Verification items for the finished model (mm, model axes). Round coordinates to 2 decimals unless told otherwise and drop trailing zeros. Loops run counter-clockwise (first coordinate to the right, second up) from the corner with the lowest first, then second, coordinate; pieces in that order, holes last. Notation, with made-up numbers: M 13.25,10 L 32.25,10 A35 cw 32.25,45 Z; hole C 25.25,-21 d10. An arc over 180 degrees is marked long. One line per item, written item: value.
Autodesk Inventor part; units mm, degrees
ref_plane "YZ Plane" through (0, 0, 0) normal (1, 0, 0) x (0, 1, 0)
ref_plane "XZ Plane" through (0, 0, 0) normal (0, 1, 0) x (-1, 0, 0)
ref_plane "XY Plane" through (0, 0, 0) normal (0, 0, 1) x (1, 0, 0)
sketch "Sketch1" plane through (0, 0, 0) normal (0, 0, 1) x (1, 0, 0)
  line L0 (-7.5, 73) -> (7.5, 73)
  line L1 (7.5, 73) -> (7.5, 70)
  line L2 (-7.5, 70) -> (-7.5, 73)
  line L3 (-40.4145, 70) -> (-7.5, 70)
  line L4 (7.5, 70) -> (40.4145, 70)
  line L5 (-66.9699, 30.0048) -> (-59.4699, 42.9952)
  line L6 (-59.4699, 42.9952) -> (-56.8718, 41.4952)
  line L7 (-64.3718, 28.5048) -> (-66.9699, 30.0048)
  line L8 (-59.4699, -42.9952) -> (-66.9699, -30.0048)
  line L9 (-66.9699, -30.0048) -> (-64.3718, -28.5048)
  line L10 (-56.8718, -41.4952) -> (-59.4699, -42.9952)
  line L11 (7.5, -73) -> (-7.5, -73)
  line L12 (-7.5, -73) -> (-7.5, -70)
  line L13 (7.5, -70) -> (7.5, -73)
  line L14 (66.9699, -30.0048) -> (59.4699, -42.9952)
  line L15 (59.4699, -42.9952) -> (56.8718, -41.4952)
  line L16 (64.3718, -28.5048) -> (66.9699, -30.0048)
  line L17 (59.4699, 42.9952) -> (66.9699, 30.0048)
  line L18 (66.9699, 30.0048) -> (64.3718, 28.5048)
  line L19 (56.8718, 41.4952) -> (59.4699, 42.9952)
  line L20 (-80.829, 0) -> (-64.3718, 28.5048)
  line L21 (-56.8718, 41.4952) -> (-40.4145, 70)
  line L22 (40.4145, 70) -> (56.8718, 41.4952)
  line L23 (64.3718, 28.5048) -> (80.829, 0)
  line L24 (80.829, 0) -> (64.3718, -28.5048)
  line L25 (56.8718, -41.4952) -> (40.4145, -70)
  line L26 (40.4145, -70) -> (7.5, -70)
  line L27 (-7.5, -70) -> (-40.4145, -70)
  line L28 (-40.4145, -70) -> (-56.8718, -41.4952)
  line L29 (-64.3718, -28.5048) -> (-80.829, 0)
  point P0 (0, 0)
  point P1 (0, 0)
  point P2 (0, 73)
  point P3 (-63.2199, 36.5)
  point P4 (-63.2199, -36.5)
  point P5 (0, -73)
  point P6 (63.2199, -36.5)
  point P7 (63.2199, 36.5)
  dimension "d1" = 3
  dimension "d3" = 15
  dimension "d6" = 360
  dimension "d8" = 140
  dimension "d9" = 146
extrude "Extrusion1" add sketch "Sketch1" along normal blind 3
properties part number "middle_space"
(1) Depth check by flat-ended pin: pin 1 Ø1 at (x, z) = (-36, 1.5) entering from +Y; pin 2 Ø1.5 at (y, z) = (71, 1) entering from -X; pin 3 Ø1.5 at (x, z) = (21.5, 2) entering from -Y. Enter the tip coordinate at first touch or a pass-through.
Completed:
pin 1: stops at y = 70
pin 2: stops at x = -7.5
pin 3: stops at y = -70
(2) Thickness scan on L1, parallel to X at y = -42, z = 1.35; L2, parallel to Y at x = -19.5, z = 2.3; L3, parallel to X at y = 44.5, z = 0.7. Record the ranges inside material, lowest first. Write a range as from..to.
Completed:
L1: x = -60.04..-57.75, -56.58..56.58, 57.75..60.04
L2: y = -70..70
L3: x = -55.14..55.14
(3) Sectioned sample at B-B on x = -16.5. Enter the section's corners in (y, z).
Completed:
outline: M -70,0 L 70,0 L 70,3 L -70,3 Z
(4) Sectioned sample at C-C on y = -39.5. Enter the section's corners in (x, z), and give its area (3 significant figures).
Completed:
outline: M -61.49,0 L 61.49,0 L 61.49,3 L -61.49,3 Z
area: 369 mm^2
